CAD build for the part. Positions are in the model's coordinates, mm. A direction names the side the tool comes from. Give positions to 0.01 mm unless a question says otherwise; leave off trailing zeros. Write each loop counter-clockwise with the first axis right and the second up, starting at its lowest first coordinate (ties: lowest second). Pieces come first, ordered by that corner, then holes. Notation, with made-up numbers: (71, -7) -> (88, -7) arc R15 cw to (88, 9) -> close; hole circle Ø7 at (48.5, -12.75). An arc over 180 degrees is marked (long way). Answer as a JSON object with one key per item and string values.
```python
from build123d import *

# Parameters (mm, degrees)
PAD_DEPTH          = 6
POCKET_DEPTH       = 3
SKETCH002_W        = 18.4
SKETCH002_H        = 20.85
POCKET001_DEPTH    = 3
SKETCH003_W        = 8.55
SKETCH003_H        = 1.65
POCKET002_DEPTH    = 3
PAD001_DEPTH       = 3
SKETCH005_W        = 127
SKETCH005_H        = 6
PAD002_DEPTH       = 3
SKETCH006_R        = 0.825
POCKET003_DEPTH    = 442.080062
POLARPATTERN_COUNT = 2


with BuildPart() as part:
    # Sketch → Pad (new body)
    with BuildSketch(Plane.XY):
        with BuildLine():
            ThreePointArc((-75, 28.5), (-103.5, 0), (-75, -28.5))
            Line((-75, -28.5), (75, -28.5))
            ThreePointArc((75, -28.5), (103.5, 0), (75, 28.5))
            Line((-75, 28.5), (75, 28.5))
        make_face()
    extrude(amount=PAD_DEPTH)

    # Sketch001 (on Face6 of Pad) → Pocket (cut)
    with BuildSketch(Plane.XY.offset(6)):
        with BuildLine():
            ThreePointArc((-62.5, 6), (-68.5, 0), (-62.5, -6))
            Line((-62.5, -6), (62.5, -6))
            ThreePointArc((62.5, -6), (68.5, 0), (62.5, 6))
            Line((-62.5, 6), (62.5, 6))
        make_face()
    extrude(amount=-POCKET_DEPTH, mode=Mode.SUBTRACT)

    # Sketch002 (on Face5 of Pocket) → Pocket001 (cut)
    with BuildSketch(Plane.XY.offset(6)):
        with Locations((0, -16.425)):
            Rectangle(SKETCH002_W, SKETCH002_H)
    extrude(amount=-POCKET001_DEPTH, mode=Mode.SUBTRACT)

    # Sketch003 (on Face5 of Pocket001) → Pocket002 (cut)
    with BuildSketch(Plane.XY.offset(6)):
        with Locations((0, -27.675)):
            Rectangle(SKETCH003_W, SKETCH003_H)
    extrude(amount=-POCKET002_DEPTH, mode=Mode.SUBTRACT)

    # Sketch004 (on Face5 of Pocket002) → Pad001 (join)
    with BuildSketch(Plane.XY.offset(6)):
        with BuildLine():
            ThreePointArc((-75, 28.5), (-103.5, 0), (-75, -28.5))
            Line((-75, -28.5), (75, -28.5))
            ThreePointArc((75, -28.5), (103.5, 0), (75, 28.5))
            Line((-75, 28.5), (75, 28.5))
        make_face()
        with BuildLine():
            ThreePointArc((-62.5, 6), (-68.5, 0), (-62.5, -6))
            Line((-62.5, -6), (62.5, -6))
            ThreePointArc((62.5, -6), (68.5, 0), (62.5, 6))
            Line((-62.5, 6), (62.5, 6))
        make_face(mode=Mode.SUBTRACT)
    extrude(amount=PAD001_DEPTH)

    # Sketch005 (on Face12 of Pad001) → Pad002 (join)
    with BuildSketch(Plane.XY.offset(9)):
        with BuildLine():
            ThreePointArc((-75, 28.5), (-103.5, 0), (-75, -28.5))
            Line((-75, -28.5), (75, -28.5))
            ThreePointArc((75, -28.5), (103.5, 0), (75, 28.5))
            Line((-75, 28.5), (75, 28.5))
        make_face()
        Rectangle(SKETCH005_W, SKETCH005_H, mode=Mode.SUBTRACT)
    extrude(amount=PAD002_DEPTH)

    # Sketch006 (on Face20 of Pad002) → Pocket003 (cut, through all)
    with BuildSketch(Plane.XY.offset(12)):
        with Locations((-87.5, 0)):
            Circle(SKETCH006_R)
    pocket003 = extrude(amount=-POCKET003_DEPTH, mode=Mode.SUBTRACT)

    # PolarPattern: Pocket003 ×2 about axis
    polarpattern_axis = Axis((0, 0, 12), (0, 0, 1))
    for i in range(1, POLARPATTERN_COUNT):
        add(pocket003.rotate(polarpattern_axis, i * 360 / POLARPATTERN_COUNT), mode=Mode.SUBTRACT)


solid = part.part
```
1) Slice it at C-C (y = 16). List the corners of the cut face in (x, z), then the cut area to 3 significant figures.
Model answer:
{"outline": "(-98.58, 0) -> (98.58, 0) -> (98.58, 12) -> (-98.58, 12) -> close", "area": "2,370 mm2"}
2) Slice it at A-A (x = -27.5). List the corners of the cut face in (y, z), then the cut area to 3 significant figures.
Model answer:
{"outline": "(-28.5, 0) -> (28.5, 0) -> (28.5, 12) -> (3, 12) -> (3, 9) -> (6, 9) -> (6, 3) -> (-6, 3) -> (-6, 9) -> (-3, 9) -> (-3, 12) -> (-28.5, 12) -> close", "area": "594 mm2"}
3) Wall check: probe 1 along Y at (x, z) = (-12, 10.5); probe 2 along Y at (x, z) = (2.5, 7.25); probe 3 along Z at (x, y) = (56, -3.5). Give the ranges that are in metal, low to high.
Model answer:
{"probe 1": "y = -28.5 to -3, 3 to 28.5", "probe 2": "y = -28.5 to -6, 6 to 28.5", "probe 3": "z = 0 to 3, 9 to 12"}
4) Mould opens along Z. For faces 3 (the flat face through (0, -17, 6)), 4 (the cylindrical face through (68.5, -0.1, 6)), 5 (the flat face through (-1, -28.5, 7)), 6 (the flat face through (-1, 7, 12)) say: released by +Z, released by -Z, zero draft, split by the parting line, or undercut.
Model answer:
{"face 3": "undercut", "face 4": "undercut", "face 5": "zero draft", "face 6": "released by +Z"}
5) Slice it at B-B (y = -14.5). List the corners of the cut face in (x, z), then the cut area to 3 significant figures.
Model answer:
{"outline": "(-99.54, 0) -> (99.54, 0) -> (99.54, 12) -> (-99.54, 12) -> close; hole (-9.2, 3) -> (9.2, 3) -> (9.2, 6) -> (-9.2, 6) -> close", "area": "2,330 mm2"}
6) Pin check, flat tips, straight feed: pin 1 (1.5 mm diameter, centred on y = -16.5, z = 5, fed in from +X); pin 2 (1.5 mm diameter, centred on y = 0.5, z = 10.5, fed in from -X); pin 3 (1.5 mm diameter, centred on y = -1.5, z = 11, fed in from +X). Stop position of each tip, or through.
Model answer:
{"pin 1": "stops at x = 98.75", "pin 2": "stops at x = -103.5", "pin 3": "stops at x = 103.49"}
7) 3-axis set-ups, long thin cutter, end or side, ignore diameter. For faces 1 (the flat face through (-1, 28.5, 6)), 2 (the flat face through (-1, 4, 9)): which of +Z, -Z, +X, -X, +Y, -Y reach the whole face in a straight line?
Model answer:
{"face 1": "+Z, -Z, +X, -X, +Y", "face 2": "none"}
